The listing builds one solid part. Answer for the finished solid, in the listing's coordinates (mm). A direction names the side the tool comes from. Round coordinates to 2 decimals unless told otherwise and drop trailing zeros. Order: outer loops, then holes, each group sorted by start corner. A loop starts at its lowest first (then second) coordinate and runs counter-clockwise, first axis right, second up. Notation, with made-up numbers: (29, 58.25) -> (81, 58.25) arc R25 ccw to (81, 79.25) -> close; hole circle Ø4 at (-17.75, 58). An arc over 180 degrees is marked (long way). Answer in a Markdown table with one row per item. Add a question column.
```python
from build123d import *

# Parameters (mm, degrees)
F0_W     = 60
F0_H     = 60
F1_DEPTH = 32
F3_DEPTH = 48
F5_DEPTH = 32
F6_W     = 30
F6_H     = 17
F7_DEPTH = 60


with BuildPart() as f1:
    # F0 (on Top) → F1 (new body)
    with BuildSketch(Plane.XY):
        Rectangle(F0_W, F0_H)
    extrude(amount=F1_DEPTH)

    # F2 (on face) → F3 (join)
    with BuildSketch(Plane.XY.offset(32)):
        with BuildLine():
            Line((15.811388, 7.5), (21.213203, 7.5))
            ThreePointArc((21.213203, 7.5), (0, 22.5), (-21.213203, 7.5))
            Line((-21.213203, 7.5), (-15.811388, 7.5))
            ThreePointArc((-15.811388, 7.5), (0, 17.5), (15.811388, 7.5))
        make_face()
        with BuildLine():
            ThreePointArc((15.811388, -7.5), (0, -17.5), (-15.811388, -7.5))
            Line((-15.811388, -7.5), (-21.213203, -7.5))
            ThreePointArc((-21.213203, -7.5), (0, -22.5), (21.213203, -7.5))
            Line((21.213203, -7.5), (15.811388, -7.5))
        make_face()
    extrude(amount=F3_DEPTH)

    # F4 (on face) → F5 (cut)
    with BuildSketch(Plane.XY.offset(32)):
        with BuildLine():
            ThreePointArc((15.811388, -7.5), (17.072629, -3.843872), (17.5, 0))
            ThreePointArc((17.5, 0), (17.072629, 3.843872), (15.811388, 7.5))
            ThreePointArc((15.811388, 7.5), (0, 17.5), (-15.811388, 7.5))
            ThreePointArc((-15.811388, 7.5), (-17.5, 0), (-15.811388, -7.5))
            ThreePointArc((-15.811388, -7.5), (0, -17.5), (15.811388, -7.5))
        make_face()
    extrude(amount=-F5_DEPTH, mode=Mode.SUBTRACT)

    # F6 (on face) → F7 (cut)
    with BuildSketch(Plane.XZ.offset(30)):
        with Locations((0, 8.5)):
            Rectangle(F6_W, F6_H)
    extrude(amount=-F7_DEPTH, mode=Mode.SUBTRACT)


solid = f1.part
```
Item 1: For a pull along X with two mould halves and no side action, classify faces 1 (the face through (-30, 0, 16)), 2 (the face through (0.388, 22.497, 55.664)), 3 (the face through (-23, 0, 0)), 4 (the face through (-15, 19, 8)) as released by +X, released by -X, zero draft, split by the parting line, or undercut.
Item 2: Flat-ended cylindrical pins translate along their axes: P1, Ø10, axis at y = -11, z = 59, coming from the +X side; P2, Ø6, axis at x = -19.5, z = 63, coming from the +Y side; P3, Ø6, axis at y = -14.5, z = 36.5, coming from the -X side; P4, Ø6, axis at x = 22, y = 7, coming from the -Z side. Find the tip coordinate at first contact, or state that the pin passes through.
Item 3: The part is cut by section B-B, the plane x = -3.5. Give the vertices of the cut face in (y, z).
Item 4: A tool of negligible diameter and unlimited length cuts with its end or side. For faces 5 (the face through (0, -18, 80)), 6 (the face through (-18, -7.5, 56)), 7 (the face through (15, -20, 8)), from which of +Z, -Z, +X, -X, +Y, -Y can it reach the whole face along a straight path? Write none if from no direction.
Item 5: The part is cut by section C-C, the plane y = 3.5. Give the vertices of the cut face in (x, z).
Item 6: The part is cut by section A-A, the plane z = 5.5. Give the vertices of the cut face in (x, y), and give its area (3 significant figures).
Item 7: Find the intervals of material crossed by probe 1 along Z at (x, y) = (21, 25); probe 2 along Y at (x, z) = (-6, 19); probe 3 along X at (y, z) = (5, 27.5), in increasing order. Write a range as [from, to].
Item 8: The part is cut by section D-D, the plane z = 65. Give the vertices of the cut face in (x, y), and give its area (3 significant figures).
Resolved:
| question | item | result |
|---|---|---|
| 1 | face 1 | released by -X |
| 1 | face 2 | split by the parting line |
| 1 | face 3 | zero draft |
| 1 | face 4 | undercut |
| 2 | P1 | x = 21.21 |
| 2 | P2 | y = 15.3 |
| 2 | P3 | x = -19.34 |
| 2 | P4 | z = 0 |
| 3 | outline | (-30, 17) -> (-17.15, 17) -> (-17.15, 80) -> (-22.23, 80) -> (-22.23, 32) -> (-30, 32) -> close; (17.15, 17) -> (30, 17) -> (30, 32) -> (22.23, 32) -> (22.23, 80) -> (17.15, 80) -> close |
| 4 | face 5 | +Z, +X, -X, +Y, -Y |
| 4 | face 6 | +Z, +X, -X |
| 4 | face 7 | -Z, +Y, -Y |
| 5 | outline | (-30, 0) -> (-17.15, 0) -> (-17.15, 32) -> (-30, 32) -> close; (17.15, 0) -> (30, 0) -> (30, 32) -> (17.15, 32) -> close |
| 6 | outline | (-30, -30) -> (-15, -30) -> (-15, -9.01) arc R17.5 cw to (-15.81, -7.5) arc R17.5 cw to (-15.81, 7.5) arc R17.5 cw to (-15, 9.01) -> (-15, 30) -> (-30, 30) -> close; (15, -30) -> (30, -30) -> (30, 30) -> (15, 30) -> (15, 9.01) arc R17.5 cw to (15.81, 7.5) arc R17.5 cw to (17.5, 0) arc R17.5 cw to (15.81, -7.5) arc R17.5 cw to (15, -9.01) -> close |
| 6 | area | 1,740 mm2 |
| 7 | probe 1 | [0, 32] |
| 7 | probe 2 | [-30, -16.44], [16.44, 30] |
| 7 | probe 3 | [-30, -16.77], [16.77, 30] |
| 8 | outline | (-21.21, -7.5) arc R22.5 ccw to (21.21, -7.5) -> (15.81, -7.5) arc R17.5 cw to (-15.81, -7.5) -> close; (-21.21, 7.5) -> (-15.81, 7.5) arc R17.5 cw to (15.81, 7.5) -> (21.21, 7.5) arc R22.5 ccw to start |
| 8 | area | 474 mm2 |
